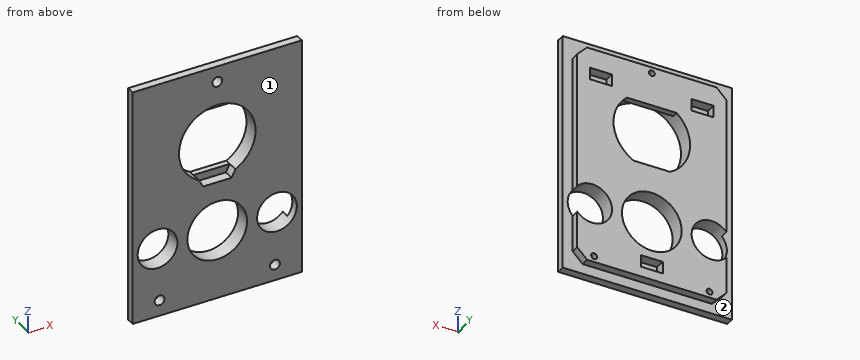
Solid Edge part; units mm, degrees
sketch "Sketch1" plane through (0, 0, 0) normal (0, -1, 0) x (1, 0, 0)
  line L0 (-42.5, -60) -> (42.5, -60)
  line L1 (42.5, -60) -> (42.5, 60)
  line L2 (42.5, 60) -> (-42.5, 60)
  line L3 (-42.5, 60) -> (-42.5, -60)
  dimension "D1" = 42.5
  dimension "D2" = 42.5
extrude "Protrusion1" add sketch "Sketch1" against normal blind 8
sketch "Sketch2" plane through (0, 0, 0) normal (0, -1, 0) x (1, 0, 0)
  arc A0 (-9.1247, 3.8) -> (9.1247, 3.8) centre (0, 20.75) cw
  line L0 (7.15, 0) -> (9.1247, 3.8)
  line L1 (-7.15, 0) -> (7.15, 0)
  line L2 (-9.1247, 3.8) -> (-7.15, 0)
  dimension "D1" = 7.15
extrude "display_cut_1" cut sketch "Sketch2" against normal blind 5
sketch "Sketch3" plane through (0, 5, 10) normal (0, -1, 0) x (1, 0, 0)
  arc A0 (12.5, 25.3894) -> (9.1247, -6.2) centre (0, 10.75) cw
  line L0 (-9.1247, -6.2) -> (9.1247, -6.2)
  arc A1 (-12.5, 25.3894) -> (-9.1247, -6.2) centre (0, 10.75) ccw
  line L1 (-12.5, 25.3894) -> (12.5, 25.3894)
  dimension "D1" = 12.5
extrude "Cutout1" cut sketch "Sketch3" against normal through all
sketch "Sketch4" plane through (0, 0, 0) normal (0, -1, 0) x (1, 0, 0)
  circle A0 centre (0, -25) radius 15
  circle A1 centre (-30, -25) radius 10
  circle A2 centre (30, -25) radius 10
extrude "Cutout2" cut sketch "Sketch4" against normal through all
sketch "Sketch5" plane through (0, 8, 0) normal (0, 1, 0) x (-1, 0, 0)
  line L0 (-5.5, -44) -> (5.5, -44)
  line L1 (5.5, -44) -> (5.5, -50)
  line L2 (5.5, -50) -> (-5.5, -50)
  line L3 (-5.5, -50) -> (-5.5, -44)
  line L4 (-31, 45) -> (-20, 45)
  line L5 (-20, 45) -> (-20, 39)
  line L6 (-20, 39) -> (-31, 39)
  line L7 (-31, 39) -> (-31, 45)
  line L8 (20, 45) -> (31, 45)
  line L9 (31, 45) -> (31, 39)
  line L10 (31, 39) -> (20, 39)
  line L11 (20, 39) -> (20, 45)
extrude "GY_521" cut sketch "Sketch5" against normal blind 5
sketch "Sketch6" plane through (0, 8, 0) normal (0, 1, 0) x (-1, 0, 0)
  line L0 (-37.5, -55) -> (37.5, -55)
  line L1 (37.5, -55) -> (37.5, 55)
  line L2 (37.5, 55) -> (-37.5, 55)
  line L3 (-37.5, 55) -> (-37.5, -55)
extrude "Extrusionsausschnitt_6" cut sketch "Sketch6" against normal blind 4 flip side to cut
chamfer "Fase_1" distance 5 angle 45 4 edges at (37.5, 6, 55) (-37.5, 6, 55) (-37.5, 6, -55) (37.5, 6, -55)
hole "Bohrung_1" at (0, 0, 52) direction (0, 1, 0) diameter 3 end up to next counterbore diameter 5 counterbore depth 5
hole "Hole1" at (-29, 0, -52) direction (0, 1, 0) diameter 3 end up to next counterbore diameter 5 counterbore depth 5
hole "Hole2" at (29, 0, -52) direction (0, 1, 0) diameter 3 end up to next counterbore diameter 5 counterbore depth 5
properties material "Nylon, allgemein"
Source: CAD feature listing. Evaluate the final solid. Frame: model axes, mm. Face numbers are marked on the shaded views. A direction names the side the tool comes from. Round coordinates to 2 decimals unless told otherwise and drop trailing zeros. Loops run counter-clockwise (first coordinate to the right, second up) from the corner with the lowest first, then second, coordinate; pieces in that order, holes last.
1. Section query D-D on z = -25. Output: boundary loops of the cut face in (x, y).
2. Ray query, L1, parallel to X at y = 2.5, z = -52; L2, parallel to Z at x = 0, y = 3.25; L3, parallel to Z at x = -30, y = 5.25. Return the intervals inside material, ascending.
3. Access query for the marked faces 1 and 2. Directions: +Z, -Z, +X, -X, +Y, -Y. A direction counts if a zero-diameter tool reaches every point of the face in a straight line with its end or side. Return the directions, or none.
4. Section query A-A on x = 0. Give the number of separate pieces and of enclosed holes in the cut face, and give its area (3 significant figures).
5. Section query B-B on z = 52. Output: boundary loops of the cut face in (x, y), and give its area (3 significant figures).
6. Contact query for flat-ended pins moving along their axis: pin 1 (2.5 mm diameter, centred on x = 0.5, z = 51, fed in from -Y); pin 2 (3.5 mm diameter, centred on x = -1, y = 7, fed in from +Z); pin 3 (4.5 mm diameter, centred on x = 29, z = -52, fed in from +Y); pin 4 (1.5 mm diameter, centred on x = 2, y = 6.5, fed in from -Z). Output: stop coordinate, or through.
7. Section query C-C on x = 24. Output: boundary loops of the cut face in (y, z).
Answers below:
1. outline: (-42.5, 0) - (-40, 0) - (-40, 4) - (-42.5, 4) - close; (-20, 0) - (-15, 0) - (-15, 8) - (-20, 8) - close; (15, 0) - (20, 0) - (20, 8) - (15, 8) - close; (40, 0) - (42.5, 0) - (42.5, 4) - (40, 4) - close
2. L1: x = -42.5 to -31.5, -26.5 to 26.5, 31.5 to 42.5
2. L2: z = -60 to -50, -44 to -40, -10 to 0, 40 to 49.5, 54.5 to 60
2. L3: z = -55 to -53.12, -50.88 to -35, -15 to 39, 45 to 55
3. face 1: +Z, -Z, +X, -X, -Y
3. face 2: +Y
4. separate pieces: 4
4. enclosed holes: 0
4. area: 321 mm2
5. outline: (-42.5, 0) - (-2.5, 0) - (-2.5, 5) - (-1.5, 5) - (-1.5, 8) - (-35.5, 8) - (-35.5, 4) - (-42.5, 4) - close; (1.5, 5) - (2.5, 5) - (2.5, 0) - (42.5, 0) - (42.5, 4) - (35.5, 4) - (35.5, 8) - (1.5, 8) - close
5. area: 590 mm2
6. pin 1: stops at y = 5
6. pin 2: stops at z = 55
6. pin 3: stops at y = 8
6. pin 4: stops at z = -55
7. outline: (0, -60) - (4, -60) - (4, -55) - (8, -55) - (8, -33) - (0, -33) - close; (0, -17) - (8, -17) - (8, 39) - (3, 39) - (3, 45) - (8, 45) - (8, 55) - (4, 55) - (4, 60) - (0, 60) - close
